Geometry: final body of the model. Coordinates: model frame, mm. Face numbers are marked on the shaded views. A direction names the side the tool comes from. Coordinates: 2 decimals unless noted, no trailing zeros. Write each loop counter-clockwise with the first axis right and the second up, starting at its lowest first coordinate (ties: lowest second). Pieces come first, ordered by that corner, then holes.
from build123d import *

# Parameters (mm, degrees)
GEAR_BOX_DEPTH      = 6.86
GEAR_BOX_DEPTH_BACK = 6.86
MOTOR_DEPTH         = 5.715
MOTOR_DEPTH_BACK    = 5.715
SKETCH2_W           = 13.61
SKETCH2_H           = 22.86
SKETCH3_R           = 1.51
SKETCH3_R_2         = 3.645
SKETCH3_R_3         = 2.43
SPACER_DEPTH        = 0.45
SPACER_BACK_START   = 0.45
SKETCH5_R           = 3.645
SKETCH5_R_2         = 2.43
SPACER_BACK_DEPTH   = 0.45
SKETCH4_R           = 1.095
OUTPUT_SHAFT_DEPTH  = 8.76


with BuildPart() as part:
    # Sketch1 → Gear Box (new, two sides: drawn at the far end of the back side and taken through both)
    with BuildSketch(Plane(origin=(0, 0, 0), x_dir=(1, 0, 0), z_dir=(0, 1, 0)).offset(-GEAR_BOX_DEPTH_BACK)):
        with BuildLine():
            Line((0, 9.98), (-28.425, 9.98))
            Line((-28.425, 9.98), (-28.425, 12.395))
            Line((-28.425, 12.395), (-30.84, 12.395))
            Line((-30.84, 12.395), (-30.84, -12.395))
            Line((-30.84, -12.395), (-28.425, -12.395))
            Line((-28.425, -12.395), (-28.425, -9.98))
            Line((-28.425, -9.98), (0, -9.98))
            ThreePointArc((0, -9.98), (9.98, 0), (0, 9.98))
        make_face()
    extrude(amount=GEAR_BOX_DEPTH + GEAR_BOX_DEPTH_BACK)

    # Sketch2 → Motor (add, two sides: drawn at the far end of the back side and taken through both)
    with BuildSketch(Plane(origin=(0, 0, 0), x_dir=(1, 0, 0), z_dir=(0, 1, 0)).offset(-MOTOR_DEPTH_BACK)):
        with Locations((-37.645, 0)):
            Rectangle(SKETCH2_W, SKETCH2_H)
    extrude(amount=MOTOR_DEPTH + MOTOR_DEPTH_BACK)

    # Sketch3 → Spacer (add)
    # profile 1 of 2: a face of its own
    with BuildSketch(Plane(origin=(0, 6.86, 0), x_dir=(1, 0, 0), z_dir=(0, 1, 0))):
        with Locations(Location((-9, 1.6, 0), (0, 0, 270))):
            Circle(SKETCH3_R)
    # profile 2 of 2: a face of its own
    with BuildSketch(Plane(origin=(0, 6.86, 0), x_dir=(1, 0, 0), z_dir=(0, 1, 0))):
        with Locations(Location((0, 0, 0), (0, 0, 270))):
            Circle(SKETCH3_R_2)
        with Locations(Location((0, 0, 0), (0, 0, 270))):
            Circle(SKETCH3_R_3, mode=Mode.SUBTRACT)
    extrude(amount=SPACER_DEPTH)

    # Sketch5 → Spacer(back) (add)
    with BuildSketch(Plane.XZ.offset(6.86).offset(SPACER_BACK_START)):
        with Locations(Location((0, 0, 0), (0, 0, 90))):
            Circle(SKETCH5_R)
        with Locations(Location((0, 0, 0), (0, 0, 90))):
            Circle(SKETCH5_R_2, mode=Mode.SUBTRACT)
    extrude(amount=-SPACER_BACK_DEPTH)

    # Sketch4 → Output Shaft (add)
    with BuildSketch(Plane(origin=(0, 6.86, 0), x_dir=(1, 0, 0), z_dir=(0, 1, 0))):
        with Locations(Location((0, 0, 0), (0, 0, 270))):
            Circle(SKETCH4_R)
    extrude(amount=OUTPUT_SHAFT_DEPTH)


solid = part.part
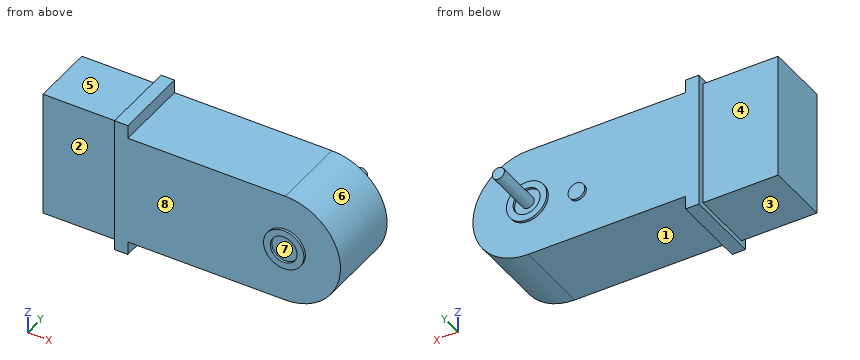
Item 1: Set-up query: the marked faces 1, 2, 3, 4 and 5. Return all of +Z, -Z, +X, -X, +Y, -Y with unobstructed straight access to the full face (end or side cutting, diameter ignored); none if empty.
Derived:
face 1: -Z, +X, +Y, -Y
face 2: +Z, -Z, -X, -Y
face 3: -Z, -X, +Y, -Y
face 4: +Z, -Z, -X, +Y
face 5: +Z, -X, +Y, -Y
Item 2: Material intervals for probe 1 along X at (y, z) = (7.1, 0) (3 decimals); probe 2 along Y at (x, z) = (-27.5, -4.5); probe 3 along X at (y, z) = (-3, 11) (3 decimals), sorted ascending.
Derived:
probe 1: x = -3.645 to -2.43, -1.095 to 1.095, 2.43 to 3.645
probe 2: y = -6.86 to 6.86
probe 3: x = -44.45 to -28.425
Item 3: Pull-direction query (X, two-part tool) for the marked faces 6, 7 and 8; classes: released by +X, released by -X, zero draft, split by the parting line, or undercut.
Derived:
face 6: released by +X
face 7: undercut
face 8: zero draft
Item 4: Section A-A, the plane x = -9. Output: boundary loops of the cut face in (y, z).
Derived:
outline: (-6.86, -9.98) - (6.86, -9.98) - (6.86, -3.11) - (7.31, -3.11) - (7.31, -0.09) - (6.86, -0.09) - (6.86, 9.98) - (-6.86, 9.98) - close
Item 5: Section B-B, the plane z = 10.5. Output: boundary loops of the cut face in (x, y) (3 decimals).
Derived:
outline: (-44.45, -5.715) - (-30.84, -5.715) - (-30.84, -6.86) - (-28.425, -6.86) - (-28.425, 6.86) - (-30.84, 6.86) - (-30.84, 5.715) - (-44.45, 5.715) - close
Item 6: Pin query (flat end, axial travel): pin 1 (8 mm diameter, centred on y = 7, z = 1, fed in from +X); pin 2 (3 mm diameter, centred on y = 9.5, z = -6.5, fed in from +X); pin 3 (2 mm diameter, centred on x = -28.5, z = -7, fed in from -Y); pin 4 (4 mm diameter, centred on x = -14, y = 1.5, fed in from -Z). Return the tip coordinate at first contact, or that it passes through.
Derived:
pin 1: stops at x = 9.98
pin 2: passes through
pin 3: stops at y = -6.86
pin 4: stops at z = -9.98
Item 7: Section C-C, the plane y = 8. Output: boundary loops of the cut face in (x, z) (3 decimals).
Derived:
outline: circle Ø2.19 at (0, 0)
Item 8: Section D-D, the plane x = -37. Output: boundary loops of the cut face in (y, z) (3 decimals), plus the area to 3 significant figures.
Derived:
outline: (-5.715, -11.43) - (5.715, -11.43) - (5.715, 11.43) - (-5.715, 11.43) - close
area: 261 mm2
